```python
from build123d import *

# Parameters (mm, degrees)
SKETCH1_R           = 6.35
BOSS_EXTRUDE2_DEPTH = 2.9972


with BuildPart() as part:
    # Sketch1 → Boss-Extrude2 (new body)
    with BuildSketch(Plane.XY):
        with BuildLine():
            Line((0, 0), (0, -9.652))
            Line((0, -9.652), (2.9972, -9.652))
            Line((2.9972, -9.652), (2.9972, -15.748))
            Line((2.9972, -15.748), (0, -15.748))
            Line((0, -15.748), (0, -22.352))
            Line((0, -22.352), (2.9972, -22.352))
            Line((2.9972, -22.352), (8.0772, -22.352))
            ThreePointArc((8.0772, -22.352), (11.1252, -25.4), (8.0772, -28.448))
            Line((8.0772, -28.448), (2.9972, -28.448))
            Line((2.9972, -28.448), (0, -28.448))
            Line((0, -28.448), (0, -35.052))
            Line((0, -35.052), (2.9972, -35.052))
            Line((2.9972, -35.052), (2.9972, -41.148))
            Line((2.9972, -41.148), (0, -41.148))
            Line((0, -41.148), (0, -47.752))
            Line((0, -47.752), (2.9972, -47.752))
            Line((2.9972, -47.752), (2.9972, -53.848))
            Line((2.9972, -53.848), (0, -53.848))
            Line((0, -53.848), (0, -60.452))
            Line((0, -60.452), (2.9972, -60.452))
            Line((2.9972, -60.452), (2.9972, -66.548))
            Line((2.9972, -66.548), (0, -66.548))
            Line((0, -66.548), (0, -73.152))
            Line((0, -73.152), (2.9972, -73.152))
            Line((2.9972, -73.152), (2.9972, -79.248))
            Line((2.9972, -79.248), (0, -79.248))
            Line((0, -79.248), (0, -85.852))
            Line((0, -85.852), (2.9972, -85.852))
            Line((2.9972, -85.852), (2.9972, -91.948))
            Line((2.9972, -91.948), (0, -91.948))
            Line((0, -91.948), (0, -98.552))
            Line((0, -98.552), (2.9972, -98.552))
            Line((2.9972, -98.552), (8.0772, -98.552))
            ThreePointArc((8.0772, -98.552), (11.1252, -101.6), (8.0772, -104.648))
            Line((8.0772, -104.648), (2.9972, -104.648))
            Line((2.9972, -104.648), (0, -104.648))
            Line((0, -104.648), (0, -111.252))
            Line((0, -111.252), (2.9972, -111.252))
            Line((2.9972, -111.252), (2.9972, -117.348))
            Line((2.9972, -117.348), (0, -117.348))
            Line((0, -117.348), (0, -127))
            Line((0, -127), (63.5, -127))
            Line((63.5, -127), (63.5, -117.348))
            Line((63.5, -117.348), (60.5028, -117.348))
            Line((60.5028, -117.348), (60.5028, -111.252))
            Line((60.5028, -111.252), (63.5, -111.252))
            Line((63.5, -111.252), (63.5, -104.648))
            Line((63.5, -104.648), (60.5028, -104.648))
            Line((60.5028, -104.648), (60.5028, -98.552))
            Line((60.5028, -98.552), (63.5, -98.552))
            Line((63.5, -98.552), (63.5, -91.948))
            Line((63.5, -91.948), (60.5028, -91.948))
            Line((60.5028, -91.948), (60.5028, -85.852))
            Line((60.5028, -85.852), (63.5, -85.852))
            Line((63.5, -85.852), (63.5, -79.248))
            Line((63.5, -79.248), (60.5028, -79.248))
            Line((60.5028, -79.248), (60.5028, -73.152))
            Line((60.5028, -73.152), (63.5, -73.152))
            Line((63.5, -73.152), (63.5, -66.548))
            Line((63.5, -66.548), (60.5028, -66.548))
            Line((60.5028, -66.548), (60.5028, -60.452))
            Line((60.5028, -60.452), (63.5, -60.452))
            Line((63.5, -60.452), (63.5, -53.848))
            Line((63.5, -53.848), (60.5028, -53.848))
            Line((60.5028, -53.848), (60.5028, -47.752))
            Line((60.5028, -47.752), (63.5, -47.752))
            Line((63.5, -47.752), (63.5, -41.148))
            Line((63.5, -41.148), (60.5028, -41.148))
            Line((60.5028, -41.148), (60.5028, -35.052))
            Line((60.5028, -35.052), (63.5, -35.052))
            Line((63.5, -35.052), (63.5, -28.448))
            Line((63.5, -28.448), (60.5028, -28.448))
            Line((60.5028, -28.448), (60.5028, -22.352))
            Line((60.5028, -22.352), (63.5, -22.352))
            Line((63.5, -22.352), (63.5, -15.748))
            Line((63.5, -15.748), (60.5028, -15.748))
            Line((60.5028, -15.748), (60.5028, -9.652))
            Line((60.5028, -9.652), (63.5, -9.652))
            Line((63.5, -9.652), (63.5, 0))
            Line((63.5, 0), (0, 0))
        make_face()
        with Locations((31.75, -63.5)):
            Circle(SKETCH1_R, mode=Mode.SUBTRACT)
    extrude(amount=BOSS_EXTRUDE2_DEPTH)


solid = part.part
```
The listing builds one solid part. Answer for the finished solid, in the listing's coordinates (mm). A direction names the side the tool comes from. Give positions to 0.01 mm unless a question says otherwise; leave off trailing zeros. Loops run counter-clockwise (first coordinate to the right, second up) from the corner with the lowest first, then second, coordinate; pieces in that order, holes last. Notation, with made-up numbers: (78.25, 38) - (109.25, 38) arc R19 ccw to (109.25, 55) - close; hole circle Ø2 at (34, 67.25). An arc over 180 degrees is marked (long way). Return JSON: item names as keys, results as strings. Group by question number.
1. Find section B-B (y = -63.5). Write down the section's boundary in (x, z).
2. Find section C-C (y = -116). Write down the section's boundary in (x, z), then the cut area to 3 significant figures.
3. Find section A-A (x = 31.75). Write down the section's boundary in (y, z), then the cut area to 3 significant figures.
4. Straight lines are drawn through the part: line 1 (Y direction, x = 9.5, z = 2.85); line 2 (Y direction, x = 6.5, z = 1); line 3 (Y direction, x = 31.75, z = 1.8). For each, find the intervals that lie inside material, in ascending order. Write a range as [from, to].
5. Which of the six approach directions +Z, -Z, +X, -X, +Y, -Y give full straight-line access (tool end or side, diameter ignored) to faces 1 (the flat face through (1, -73.152, 1)), 2 (the flat face through (60.503, -38, 1)), 3 (the flat face through (63.5, -108, 1))?
6. Determine the mould class of faces 4 (the flat face through (63.5, -83, 1)), 5 (the flat face through (2, -117.348, 1)), 6 (the flat face through (62, -117.348, 1)) for opening direction Y: pulls with the +Y half, pulls with the -Y half, needs draft (parallel to the pull), parting line crosses it, or undercut.
7. Find section D-D (y = -25.4). Write down the section's boundary in (x, z).
Verdict:
{
 "1": {"outline": "(3, 0) - (25.4, 0) - (25.4, 3) - (3, 3) - close; (38.1, 0) - (60.5, 0) - (60.5, 3) - (38.1, 3) - close"},
 "2": {"outline": "(3, 0) - (60.5, 0) - (60.5, 3) - (3, 3) - close", "area": "172 mm^2"},
 "3": {"outline": "(-127, 0) - (-69.85, 0) - (-69.85, 3) - (-127, 3) - close; (-57.15, 0) - (0, 0) - (0, 3) - (-57.15, 3) - close", "area": "343 mm^2"},
 "4": {"line 1": "y = [-127, -104.3], [-98.9, -28.1], [-22.7, 0]", "line 2": "y = [-127, -104.65], [-98.55, -28.45], [-22.35, 0]", "line 3": "y = [-127, -69.85], [-57.15, 0]"},
 "5": {"face 1": "+Z, -Z, -X", "face 2": "+Z, -Z, +X", "face 3": "+Z, -Z, +X, +Y, -Y"},
 "6": {"face 4": "needs draft", "face 5": "undercut", "face 6": "undercut"},
 "7": {"outline": "(11.13, 0) - (60.5, 0) - (60.5, 3) - (11.13, 3) - close"}
}
